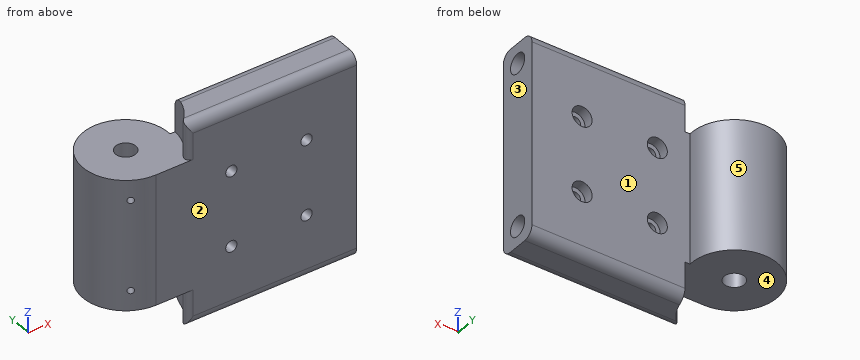
from build123d import *
from OCP.BRepFilletAPI import BRepFilletAPI_MakeFillet

# Parameters (mm, degrees)
BOSS_EXTRUDE2_DEPTH             = 40.5
SKETCH18_R                      = 19
CUT_EXTRUDE7_DEPTH              = 14.5
CUT_EXTRUDE8_REACH              = 92.73
SKETCH19_R                      = 4
SKETCH20_R                      = 3.95
CUT_EXTRUDE10_DEPTH             = 40
FILLET2_R1                      = 4
FILLET2_R2                      = 2
CBORE_FOR_M4_SHCS1_D            = 4.5
CBORE_FOR_M4_SHCS1_CBORE_D      = 8
CBORE_FOR_M4_SHCS1_CBORE_DEPTH  = 4
M3_TAPPED_HOLE1_D               = 2.5
M3_TAPPED_HOLE1_DEPTH           = 17
M3_TAPPED_HOLE1_ON_FACE_2_D     = 2.5
M3_TAPPED_HOLE1_ON_FACE_2_DEPTH = 17


with BuildPart() as part:
    # Sketch11 → Boss-Extrude2 (new body)
    with BuildSketch(Plane.XY):
        with BuildLine():
            Line((0, 0), (80, 0))
            Line((80, 0), (80, 16))
            Line((80, 16), (16.970562748, 16))
            ThreePointArc((16.970562748, 16), (-11.66190379, 29.369316877), (0, 0))
        make_face()
    boss_extrude2 = extrude(amount=-BOSS_EXTRUDE2_DEPTH)

    # Sketch18 → Cut-Extrude7 (cut)
    with BuildSketch(Plane.XY):
        with Locations((0, 17)):
            Circle(SKETCH18_R)
    cut_extrude7 = extrude(amount=-CUT_EXTRUDE7_DEPTH, mode=Mode.SUBTRACT)

    # Sketch19 → Cut-Extrude8 (cut, up to next)
    with BuildSketch(Plane.XY.offset(-14.5), mode=Mode.PRIVATE) as cut_extrude8_sk1:
        with Locations((0, 17)):
            Circle(SKETCH19_R)
    cut_extrude8_tool1 = extrude(cut_extrude8_sk1.sketch, amount=-CUT_EXTRUDE8_REACH, mode=Mode.PRIVATE) & part.part
    cut_extrude8 = cut_extrude8_tool1.solids().sort_by_distance((0, 17, -14.5))[0]
    add(cut_extrude8, mode=Mode.SUBTRACT)

    # Sketch20 → Cut-Extrude10 (cut)
    with BuildSketch(Plane(origin=(80, 0, 0), x_dir=(0, 0, -1), z_dir=(1, 0, 0))):
        with Locations((8, 8)):
            Circle(SKETCH20_R)
    cut_extrude10 = extrude(amount=-CUT_EXTRUDE10_DEPTH, mode=Mode.SUBTRACT)

    # Mirror2: Boss-Extrude2, Cut-Extrude7, Cut-Extrude8, Cut-Extrude10 across plane
    add(boss_extrude2.mirror(Plane(origin=(0, 17, -40.5), x_dir=(1, 0, 0), z_dir=(0, 0, -1))))
    add(cut_extrude7.mirror(Plane(origin=(0, 17, -40.5), x_dir=(1, 0, 0), z_dir=(0, 0, -1))), mode=Mode.SUBTRACT)
    add(cut_extrude8.mirror(Plane(origin=(0, 17, -40.5), x_dir=(1, 0, 0), z_dir=(0, 0, -1))), mode=Mode.SUBTRACT)
    add(cut_extrude10.mirror(Plane(origin=(0, 17, -40.5), x_dir=(1, 0, 0), z_dir=(0, 0, -1))), mode=Mode.SUBTRACT)

    # Fillet2: one fillet with a radius per group of edges: ONE call of the kernel's fillet builder (fillet() takes one radius for all edges)
    fillet2_edges_1 = [part.edges().sort_by_distance(p)[0] for p in [
        (44.242640687, 0, 0),
        (49.486832981, 16, -81),
        (49.486832981, 16, 0),
        (44.242640687, 0, -81),
    ]]
    fillet2_edges_2 = [part.edges().sort_by_distance(p)[0] for p in [
        (8.485281374, 0, -7.25),
        (8.485281374, 0, -73.75),
    ]]
    fillet2 = BRepFilletAPI_MakeFillet(part.part.solid().wrapped)
    for e in fillet2_edges_1:
        fillet2.Add(FILLET2_R1, e.wrapped)
    for e in fillet2_edges_2:
        fillet2.Add(FILLET2_R2, e.wrapped)
    add(Compound.cast(fillet2.Shape()), mode=Mode.REPLACE)

    # CBORE for M4 SHCS1 (through all)
    with Locations(Plane(origin=(0, 16, 0), x_dir=(1, 0, 0), z_dir=(0, 1, 0))):
        with Locations((60, 55.5), (60, 25.5), (30, 25.5), (30, 55.5)):
            CounterBoreHole(CBORE_FOR_M4_SHCS1_D / 2, CBORE_FOR_M4_SHCS1_CBORE_D / 2, CBORE_FOR_M4_SHCS1_CBORE_DEPTH)

    # M3 Tapped Hole1
    with Locations(Plane(origin=(-8.5, 2.277568136, -58.5), x_dir=(-0.866025403784, 0.5, 0), z_dir=(-0.5, -0.866025403784, 0))):
        with Locations((0, 0)):
            Hole(M3_TAPPED_HOLE1_D / 2, depth=M3_TAPPED_HOLE1_DEPTH)

    # M3 Tapped Hole1 on face 2
    with Locations(Plane(origin=(-8.5, 2.277568136, -22.5), x_dir=(-0.866025302838, 0.500000174844, 0), z_dir=(-0.500000174844, -0.866025302838, 0))):
        with Locations((0, 0)):
            Hole(M3_TAPPED_HOLE1_ON_FACE_2_D / 2, depth=M3_TAPPED_HOLE1_ON_FACE_2_DEPTH)


solid = part.part
The model under review builds one solid part; all positions refer to its coordinate system, in mm. Face numbers are marked on the shaded views. A direction names the side the tool comes from. Round coordinates to 2 decimals unless told otherwise and drop trailing zeros. Write each loop counter-clockwise with the first axis right and the second up, starting at its lowest first coordinate (ties: lowest second). Pieces come first, ordered by that corner, then holes. Notation, with made-up numbers: M -2.5,47.5 L 9.5,47.5 A22 cw 9.5,59.5 Z; hole C -39.5,12.5 d6. An arc over 180 degrees is marked long. Answer as CSV lines item,"result". Start each with the question number.
Q1. The part is to be moulded in two halves that separate along X. For the marked faces 3, 4 and 5, say which applies: +X half, -X half, draft (parallel to the pull), parting line (faces both ways), or undercut.
Q2. Tool access review of the marked faces 1 and 2: name each direction out of +Z, -Z, +X, -X, +Y, -Y from which nothing blocks a thin tool from reaching the whole face with its end or side.
Q3. Consider section C-C, the plane x = 30. Give the boundary of the cut face in (y, z).
Q4. Consider section B-B, the plane z = -25.5. Give the boundary of the cut face in (x, y).
Q5. Wall thickness on line 1 along Z through (x, y) = (60, 14.45); line 2 along X through (y, z) = (14, -55); line 3 along Z through (x, y) = (60, 7): over which ranges is each line inside the solid? List them lowest first.
Q6. Consider section D-D, the plane z = -73. Give the boundary of the cut face in (x, y), then the cut area to 3 significant figures.
Q7. Clearance check with flat-ended pins moving along their axes: P1, Ø6.5, axis at x = 60, z = -55, coming from the +Y side; P2, Ø9, axis at x = 28.5, z = -26.5, coming from the +Y side; P3, Ø8, axis at x = -6.5, z = -33.5, coming from the -Y side. State where each tip first meets the part, or that it passes through.
Q8. Consider section A-A, the plane x = 60. Give the boundary of the cut face in (y, z).
Result set:
1,face 3,"+X half"
1,face 4,"draft"
1,face 5,"parting line"
2,face 1,"+Z, -Z, +X, +Y"
2,face 2,"+Z, -Z, +X, -X, -Y"
3,outline,"M 0,-77 A4 ccw 4,-81 L 12,-81 A4 ccw 16,-77 L 16,-59.5 L 12,-59.5 L 12,-57.75 L 0,-57.75 Z; M 0,-53.25 L 12,-53.25 L 12,-51.5 L 16,-51.5 L 16,-29.5 L 12,-29.5 L 12,-27.75 L 0,-27.75 Z; M 0,-23.25 L 12,-23.25 L 12,-21.5 L 16,-21.5 L 16,-4 A4 ccw 12,0 L 4,0 A4 ccw 0,-4 Z"
4,outline,"M 0,0 L 27.75,0 L 27.75,12 L 26,12 L 26,16 L 16.97,16 A17 ccw long Z; M 32.25,0 L 57.75,0 L 57.75,12 L 56,12 L 56,16 L 34,16 L 34,12 L 32.25,12 Z; M 62.25,0 L 80,0 L 80,16 L 64,16 L 64,12 L 62.25,12 Z; hole C 0,17 d8"
5,line 1,"z = -80.16 to -59.5, -51.5 to -29.5, -21.5 to -0.84"
5,line 2,"x = -16.73 to -2.65, 2.65 to 26.03, 33.97 to 56.03, 63.97 to 80"
5,line 3,"z = -81 to -76.82, -69.18 to -57.75, -53.25 to -27.75, -23.25 to -11.82, -4.18 to 0"
6,outline,"M 13.3,3.43 A2 ccw 14.7,0 L 80,0 L 80,4.05 L 40,4.05 L 40,11.95 L 80,11.95 L 80,16 L 18.97,16 A19 cw Z"
6,area,"704 mm²"
7,P1,"stops at y = 12"
7,P2,"stops at y = 16"
7,P3,"stops at y = 0.18"
8,outline,"M 0,-77 A4 ccw 4,-81 L 12,-81 A4 ccw 16,-77 L 16,-59.5 L 12,-59.5 L 12,-57.75 L 0,-57.75 Z; M 0,-53.25 L 12,-53.25 L 12,-51.5 L 16,-51.5 L 16,-29.5 L 12,-29.5 L 12,-27.75 L 0,-27.75 Z; M 0,-23.25 L 12,-23.25 L 12,-21.5 L 16,-21.5 L 16,-4 A4 ccw 12,0 L 4,0 A4 ccw 0,-4 Z; hole C 8,-73 d7.9; hole C 8,-8 d7.9"
